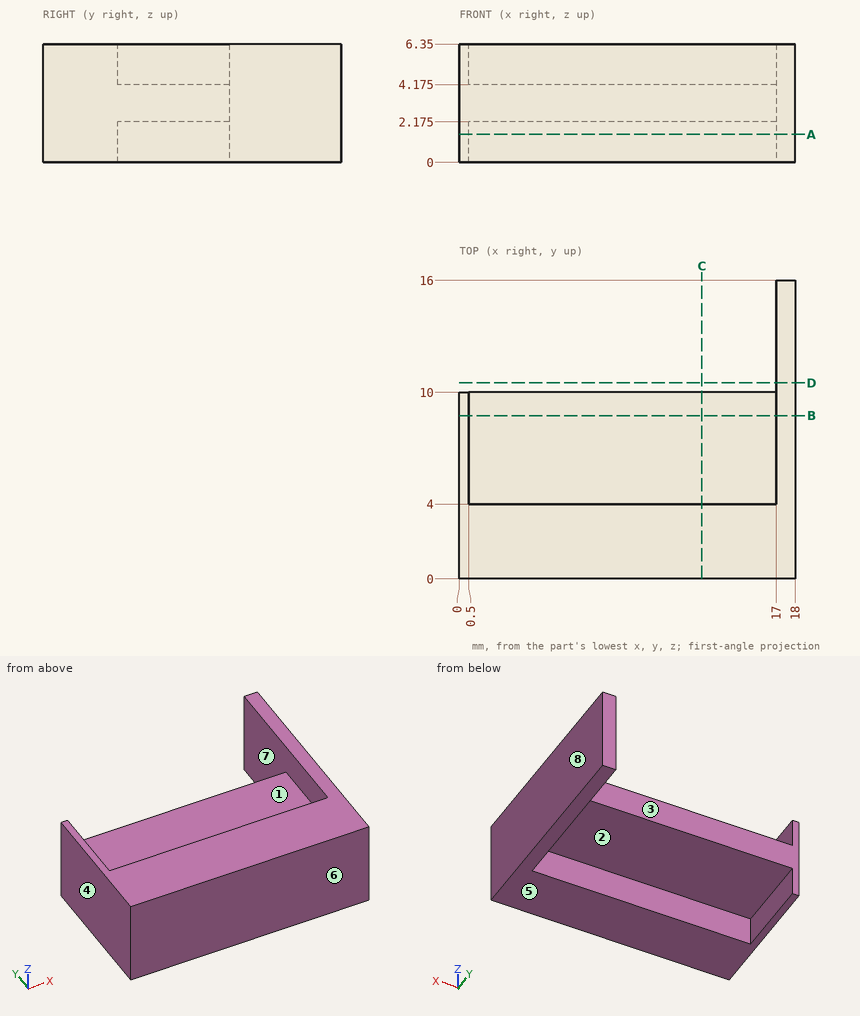
Verification items for this drawing (mm, ordinates from the low corner). A direction names the side the tool comes from. Coordinates: 2 decimals unless noted, no trailing zeros. Write each loop counter-clockwise with the first axis right and the second up, starting at its lowest first coordinate (ties: lowest second). Pieces come first, ordered by that corner, then holes. Notation, with made-up numbers: M 36.5,45.25 L 59.5,45.25 A19 cw 59.5,70.25 Z; hole C 84.5,70 d8. An arc over 180 degrees is marked long. Answer as a JSON object with one key per item and string values.
1. Section check D-D, the plane y = 10.5. Enter the section's corners in (x, z).
Answers below:
{"outline": "M 17,0 L 18,0 L 18,6.35 L 17,6.35 Z"}
2. Tool access check on the marked faces 1, 2, 3, 4 and 5. Record the directions out of +Z, -Z, +X, -X, +Y, -Y that give a thin tool (end or side, any length) a straight path to the whole face; none if there is none.
Answers below:
{"face 1": "+Z, +Y", "face 2": "-Z, +Y", "face 3": "+Z, -Z, -X, +Y", "face 4": "+Z, -Z, -X, +Y, -Y", "face 5": "-Z, +X, -X, +Y, -Y"}
3. Go/stop test with flat-tipped pins: pin 1 Ø1.7 at (x, z) = (8.5, 0.5) entering from +Y; pin 2 Ø3 at (x, y) = (6.5, 6) entering from -Z (3 decimals); pin 3 Ø6 at (x, y) = (5.5, 14.5) entering from +Z; pin 4 Ø1.9 at (x, z) = (12, 3) entering from +Y. Record where each tip stops, or that it passes through.
Answers below:
{"pin 1": "stops at y = 4", "pin 2": "stops at z = 2.175", "pin 3": "passes through", "pin 4": "stops at y = 10"}
4. Scan lines: L1, parallel to X at y = 8.75, z = 4.25; L2, parallel to Y at x = 9.5, z = 3; L3, parallel to X at y = 12, z = 1.25. Record each from-to range of solid material in increasing order.
Answers below:
{"L1": "x = 0 to 0.5, 17 to 18", "L2": "y = 0 to 10", "L3": "x = 17 to 18"}
5. Draft check along X on the marked faces 6, 7 and 8. Enter one of: released by +X, released by -X, zero draft, split by the parting line, or undercut.
Answers below:
{"face 6": "zero draft", "face 7": "undercut", "face 8": "released by +X"}
6. Section check B-B, the plane y = 8.75. Enter the section's corners in (x, z) (3 decimals), plus the area to 3 significant figures.
Answers below:
{"outline": "M 0,0 L 0.5,0 L 0.5,2.175 L 17,2.175 L 17,0 L 18,0 L 18,6.35 L 17,6.35 L 17,4.175 L 0.5,4.175 L 0.5,6.35 L 0,6.35 Z", "area": "42.5 mm²"}
7. Section check C-C, the plane x = 13. Enter the section's corners in (y, z) (3 decimals), plus the area to 3 significant figures.
Answers below:
{"outline": "M 0,0 L 4,0 L 4,2.175 L 10,2.175 L 10,4.175 L 4,4.175 L 4,6.35 L 0,6.35 Z", "area": "37.4 mm²"}
8. Section check A-A, the plane z = 1.5. Enter the section's corners in (x, y), plus the area to 3 significant figures.
Answers below:
{"outline": "M 0,0 L 18,0 L 18,16 L 17,16 L 17,4 L 0.5,4 L 0.5,10 L 0,10 Z", "area": "87.0 mm²"}
